CAD build for the part. Positions are in the model's coordinates, mm. Face numbers are marked on the shaded views. Round coordinates to 2 decimals unless told otherwise and drop trailing zeros. Loops run counter-clockwise (first coordinate to the right, second up) from the corner with the lowest first, then second, coordinate; pieces in that order, holes last. Notation, with made-up numbers: M 77,70.5 L 135,70.5 A32 ccw 135,108.5 Z; hole C 41,-9 d1. An arc over 180 degrees is marked long. Use a Markdown table: item, result. Add a question column.
(1) Band-saw the part on B-B, the plane z = 0. Write the cut outline in (x, y), and give its area (4 significant figures).
(2) Band-saw the part on A-A, the plane y = 27. Write the cut outline in (x, z) (3 decimals).
(3) Flat gauge pins, fed straight in: P1, Ø1.5, axis at x = 2, y = 17.5, coming from the -Z side; P2, Ø1.5, axis at x = 3, z = 2, coming from the +Y side. Where does each tip first touch, or does it go through?
(4) Wall check: L1, parallel to X at y = 32.25, z = 0; L2, parallel to Y at x = 1, z = 3.25; L3, parallel to X at y = 33, z = 0.5. Give the ranges that are in metal, low to high.
(5) Two-plate mould, pull along X, no slides. Class the marked faces 1 and 2: released by +X, released by -X, zero draft, split by the parting line, or undercut.
(6) Band-saw the part on C-C, the plane y = 14. Write the cut outline in (x, z), and give its area (3 significant figures).
from build123d import *

# Parameters (mm, degrees)
CROQUIS1_R              = 4
SALIENTE_EXTRUIR1_DEPTH = 25
CROQUIS2_R              = 2.5
SALIENTE_EXTRUIR2_DEPTH = 10
CHAFL_N1_SIZE           = 0.5
CHAFL_N2_SIZE           = 0.5


with BuildPart() as part:
    # Croquis1 → Saliente-Extruir1 (new body)
    with BuildSketch(Plane(origin=(0, 0, 0), x_dir=(1, 0, 0), z_dir=(0, 1, 0))):
        with Locations(Location((0, 0, 0), (0, 0, 270))):
            Circle(CROQUIS1_R)
    extrude(amount=SALIENTE_EXTRUIR1_DEPTH)

    # Croquis2 → Saliente-Extruir2 (add)
    with BuildSketch(Plane(origin=(0, 25, 0), x_dir=(1, 0, 0), z_dir=(0, 1, 0))):
        with Locations(Location((0, 0, 0), (0, 0, 270))):
            Circle(CROQUIS2_R)
        with BuildLine():
            Line((-0.175, 1.489756692), (-0.175, 1.697953702))
            Line((-0.175, 1.697953702), (0.175, 1.697953702))
            Line((0.175, 1.697953702), (0.175, 1.489756692))
            ThreePointArc((0.175, 1.489756692), (0, -1.5), (-0.175, 1.489756692))
        make_face(mode=Mode.SUBTRACT)
    extrude(amount=SALIENTE_EXTRUIR2_DEPTH)

    # Chaflán1
    chafl_n1_edges = [part.edges().sort_by_distance(p)[0] for p in [
        (0, 25, -4),
    ]]
    chamfer(chafl_n1_edges, length=CHAFL_N1_SIZE)

    # Chaflán2
    chafl_n2_edges = [part.edges().sort_by_distance(p)[0] for p in [
        (0, 0, -4),
    ]]
    chamfer(chafl_n2_edges, length=CHAFL_N2_SIZE)


solid = part.part
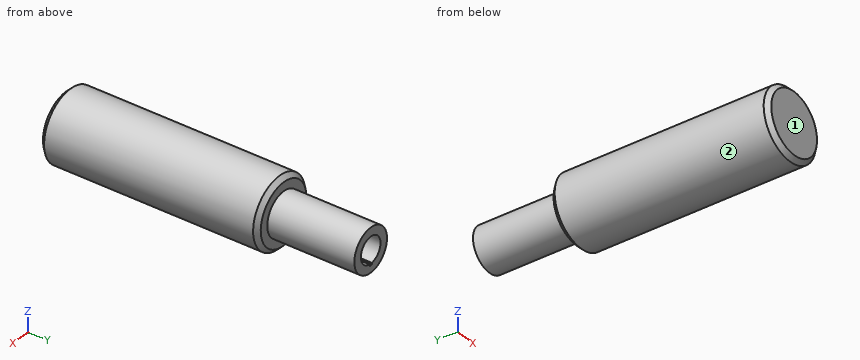
Return value:
| question | item | result |
|---|---|---|
| 1 | outline | M -4,0.5 L -3.5,0 L 3.5,0 L 4,0.5 L 4,24.5 L 3.5,25 L 2.5,25 L 2.5,35 L 1.5,35 L 1.5,25 L -1.5,25 L -1.5,35 L -2.5,35 L -2.5,25 L -3.5,25 L -4,24.5 Z |
| 1 | area | 219.5 mm^2 |
| 2 | outline | C 0,0 d5; hole M -0.175,-1.698 L 0.175,-1.698 L 0.175,-1.49 A1.5 ccw long -0.175,-1.49 Z |
| 3 | P1 | z = -3.8 |
| 3 | P2 | y = 25 |
| 4 | L1 | -2.5 to -1.5, 1.5 to 2.5 |
| 4 | L2 | 0 to 25 |
| 4 | L3 | -2.45 to -1.41, 1.41 to 2.45 |
| 5 | face 1 | zero draft |
| 5 | face 2 | split by the parting line |
| 6 | outline | C 0,0 d8 |
| 6 | area | 50.3 mm^2 |
